```python
from build123d import *

# Parameters (mm, degrees)
SKETCH008_W       = 164
SKETCH008_H       = 60
PAD003_DEPTH      = 2.5
PAD003_DEPTH_BACK = 2.95
SKETCH009_W       = 163.52
SKETCH009_H       = 59.52
POCKET005_DEPTH   = 3
POCKET005_TAPER   = 25
PAD004_DEPTH      = 4.9
PAD004_DEPTH_BACK = 4.9
PAD005_DEPTH      = 4.9
PAD005_DEPTH_BACK = 4.9
SKETCH012_W       = 9.35
SKETCH012_H       = 33.56
SKETCH012_W_2     = 6.6
SKETCH012_H_2     = 6.6
POCKET006_DEPTH   = 2.45


with BuildPart() as part:
    # Sketch008 (on ShapeBinder) → Pad003 (new body, two sides)
    with BuildSketch(Plane.XY.offset(20.89)) as pad003_sk:
        Rectangle(SKETCH008_W, SKETCH008_H)
    extrude(amount=PAD003_DEPTH)
    extrude(pad003_sk.sketch, amount=-PAD003_DEPTH_BACK)

    # Sketch009 (on Face5 of Pad003) → Pocket005 (cut)
    with BuildSketch(Plane(origin=(0, 0, 17.94), x_dir=(1, 0, 0), z_dir=(0, 0, -1))):
        Rectangle(SKETCH009_W, SKETCH009_H)
    extrude(amount=-POCKET005_DEPTH, taper=POCKET005_TAPER, mode=Mode.SUBTRACT)

    # Sketch010 → Pad004 (join, two sides)
    with BuildSketch(Plane.YZ) as pad004_sk:
        with BuildLine():
            Line((-27.5, 20.94), (-28.5, 20.94))
            Line((-28.5, 20.94), (-28.5, 16.423975))
            ThreePointArc((-28.745041, 16.082391), (-28.58568, 16.226755), (-28.5, 16.423975))
            ThreePointArc((-28.745041, 16.082391), (-28.97303, 15.529737), (-28.497162, 15.167859))
            Line((-28.497162, 15.167859), (-27.5, 15.167859))
            Line((-27.5, 20.94), (-27.5, 15.167859))
        make_face()
        with BuildLine():
            Line((27.5, 20.94), (28.5, 20.94))
            Line((28.5, 20.94), (28.5, 16.423975))
            ThreePointArc((28.5, 16.423975), (28.58568, 16.226755), (28.745041, 16.082391))
            ThreePointArc((28.497162, 15.167859), (28.97303, 15.529737), (28.745041, 16.082391))
            Line((28.497162, 15.167859), (27.5, 15.167859))
            Line((27.5, 20.94), (27.5, 15.167859))
        make_face()
    extrude(amount=PAD004_DEPTH)
    extrude(pad004_sk.sketch, amount=-PAD004_DEPTH_BACK)

    # Sketch011 → Pad005 (join, two sides)
    with BuildSketch(Plane.XZ) as pad005_sk:
        with BuildLine():
            Line((-79.5, 20.94), (-80.534817, 20.94))
            Line((-80.534817, 20.94), (-80.534817, 16.445032))
            ThreePointArc((-80.76226, 16.114088), (-80.614588, 16.256228), (-80.534817, 16.445032))
            ThreePointArc((-80.76226, 16.114088), (-80.970904, 15.564248), (-80.501498, 15.209968))
            Line((-80.501498, 15.209968), (-79.5, 15.209968))
            Line((-79.5, 20.94), (-79.5, 15.209968))
        make_face()
        with BuildLine():
            Line((79.5, 20.94), (80.534817, 20.94))
            Line((80.534817, 20.94), (80.534817, 16.445032))
            ThreePointArc((80.534817, 16.445032), (80.614588, 16.256228), (80.76226, 16.114088))
            ThreePointArc((80.501498, 15.209968), (80.970904, 15.564248), (80.76226, 16.114088))
            Line((80.501498, 15.209968), (79.5, 15.209968))
            Line((79.5, 20.94), (79.5, 15.209968))
        make_face()
    extrude(amount=PAD005_DEPTH)
    extrude(pad005_sk.sketch, amount=-PAD005_DEPTH_BACK)

    # Sketch012 (on Face5 of Pad005) → Pocket006 (cut)
    with BuildSketch(Plane.XY.offset(23.39)):
        with Locations((-43.4, -0.22)):
            Rectangle(SKETCH012_W, SKETCH012_H)
        with Locations((58, 16.25)):
            Rectangle(SKETCH012_W_2, SKETCH012_H_2)
    extrude(amount=-POCKET006_DEPTH, mode=Mode.SUBTRACT)


solid = part.part
```
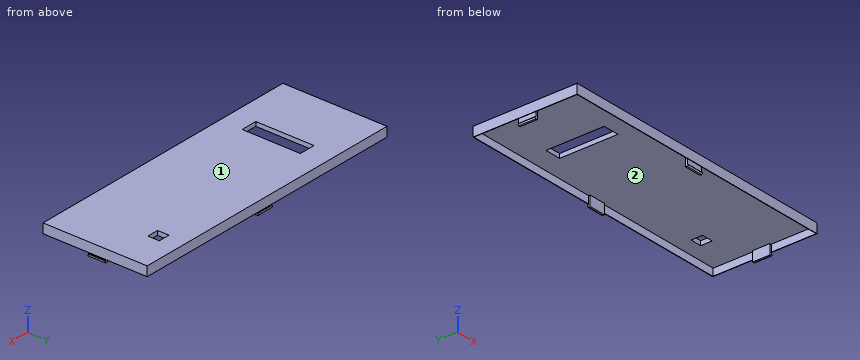
Here's how the part is built. I have some questions about the finished solid (model axes, mm). Face numbers are marked on the shaded views. Round coordinates to 2 decimals unless told otherwise and drop trailing zeros. Answer as CSV lines item,"result". Start each with the question number.
1. If we mould it in two halves opening along Y, with no side actions, what happens to the marked faces 1 and 2? For each: pulls with the +Y half, pulls with the -Y half, needs draft (parallel to the pull), parting line crosses it, or undercut.
2. I'm going to push flat-ended pins straight in: P1, Ø4.5, axis at y = -0.5, z = 17, coming from the -X side; P2, Ø1, axis at y = -12.5, z = 17, coming from the -X side; P3, Ø10, axis at x = -20, y = -16.5, coming from the -Z side; P4, Ø0.5, axis at x = -80, y = 0, coming from the -Z side. Where does each tip first touch, or does it pass through?
3. I need wall thicknesses on probe 1 along X at (y, z) = (4, 18); probe 2 along X at (y, z) = (0, 16.75); probe 3 along X at (y, z) = (8.5, 23) (3 decimals). Which ranges of each line are inside material? Lowest first, please. Write a range as from..to.
Solution:
1,face 1,"needs draft"
1,face 2,"undercut"
2,P1,"x = -82"
2,P2,"through"
2,P3,"z = 20.94"
2,P4,"z = 15.21"
3,probe 1,"-82..-81.73, -80.53..-79.5, 79.5..80.53, 81.73..82"
3,probe 2,"-80.53..-79.5, 79.5..80.53"
3,probe 3,"-82..-48.075, -38.725..82"
